Here's how the part is built. I have some questions about the finished solid (model axes, mm). Face numbers are marked on the shaded views. A direction names the side the tool comes from. Round coordinates to 2 decimals unless told otherwise and drop trailing zeros. Order: outer loops, then holes, each group sorted by start corner. A loop starts at its lowest first (then second) coordinate and runs counter-clockwise, first axis right, second up. Notation, with made-up numbers: (50, 66.5) -> (73, 66.5) arc R23 cw to (73, 96.5) -> close; hole circle Ø7 at (48, 18). An arc over 180 degrees is marked (long way). One line per item, written item: value.
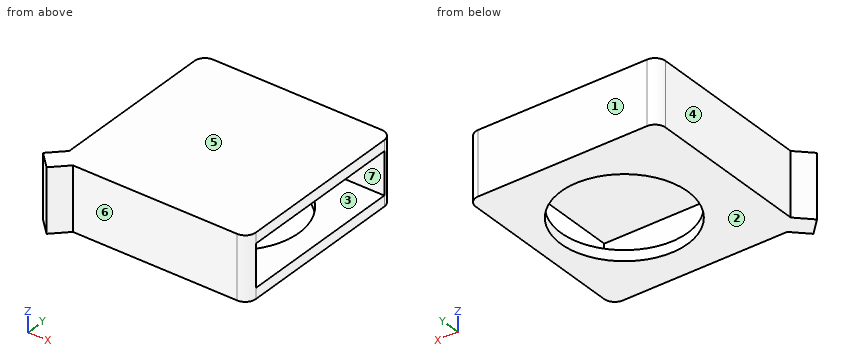
```python
from build123d import *

# Parameters (mm, degrees)
SKETCH_1_W          = 9
SKETCH_1_H          = 9
EXTRUDE_1_DEPTH     = 3
FILLET_1_R          = 0.5
SKETCH_2_R          = 3
CUT_EXTRUDE_1_DEPTH = 2.5
SKETCH_3_W          = 2
SKETCH_3_H          = 8
CUT_EXTRUDE_2_DEPTH = 8.5
EXTRUDE_2_DEPTH     = 3


with BuildPart() as part:
    # 草图1 → 凸台-拉伸1 (new body)
    with BuildSketch(Plane.XY):
        with Locations((0.284053156, -1.823920266)):
            Rectangle(SKETCH_1_W, SKETCH_1_H)
    extrude(amount=EXTRUDE_1_DEPTH)

    # 圆角1
    fillet_1_edges = [part.edges().sort_by_distance(p)[0] for p in [
        (-4.215946844, 2.676079734, 1.5),
        (4.784053156, 2.676079734, 1.5),
        (4.784053156, -6.323920266, 1.5),
        (-4.215946844, -6.323920266, 1.5),
    ]]
    fillet(fillet_1_edges, radius=FILLET_1_R)

    # 草图2 → 切除-拉伸1 (cut)
    with BuildSketch(Plane(origin=(0, 0, 0), x_dir=(-1, 0, 0), z_dir=(0, 0, -1))):
        with Locations((-0.784053156, -1.823920266)):
            Circle(SKETCH_2_R)
    extrude(amount=-CUT_EXTRUDE_1_DEPTH, mode=Mode.SUBTRACT)

    # 草图3 → 切除-拉伸2 (cut)
    with BuildSketch(Plane(origin=(4.784053156, 0, 0), x_dir=(0, 0, -1), z_dir=(1, 0, 0))):
        with Locations((-1.5, -1.823920266)):
            Rectangle(SKETCH_3_W, SKETCH_3_H)
    extrude(amount=-CUT_EXTRUDE_2_DEPTH, mode=Mode.SUBTRACT)

    # 草图4 → 凸台-拉伸2 (add)
    with BuildSketch(Plane(origin=(0, 0, 0), x_dir=(-1, 0, 0), z_dir=(0, 0, -1))):
        Polygon((4.215946844, -5.616813485), (3.508840063, -6.323920266), (4.215946844, -7.031027047), (4.923053625, -6.323920266), align=None)
    extrude(amount=-EXTRUDE_2_DEPTH)


solid = part.part
```
Q1. I want a section at D-D on x = 2. Write out the boundary of the cut face in (y, z).
Answers:
outline: (-6.32, 0) -> (-4.57, 0) -> (-4.57, 0.5) -> (-5.82, 0.5) -> (-5.82, 2.5) -> (2.18, 2.5) -> (2.18, 0.5) -> (0.92, 0.5) -> (0.92, 0) -> (2.68, 0) -> (2.68, 3) -> (-6.32, 3) -> close
Q2. I want a section at C-C on y = -1.25. Write out the boundary of the cut face in (x, z).
Answers:
outline: (-4.22, 0) -> (-2.16, 0) -> (-2.16, 0.5) -> (-3.72, 0.5) -> (-3.72, 2.5) -> (4.78, 2.5) -> (4.78, 3) -> (-4.22, 3) -> close; (3.73, 0) -> (4.78, 0) -> (4.78, 0.5) -> (3.73, 0.5) -> close
Q3. For P1, Ø0.6, axis at y = -3, z = 1.5, coming from the +X side; P2, Ø0.9, axis at x = 0.5, z = 2, coming from the -Y side, each with a flat end and sliding along its axis, tell me the tip position at first contact or that it passes through.
Answers:
P1: x = -3.72
P2: y = -6.32
Q4. Which directions (+Z, -Z, +X, -X, +Y, -Y) give clear straight access to the entire face, cutting with the end or side of a thin tool? Please do the marked faces 4, 5, 6 and 7.
Answers:
face 4: +Z, -Z, -X, +Y
face 5: +Z, +X, -X, +Y, -Y
face 6: +Z, -Z, +X, -Y
face 7: +X
Q5. I want a section at B-B on z = 2.1. Write out the boundary of the cut face in (x, y).
Answers:
outline: (-4.92, -6.32) -> (-4.22, -7.03) -> (-3.51, -6.32) -> (4.28, -6.32) arc R0.5 ccw to (4.78, -5.82) -> (-3.72, -5.82) -> (-3.72, 2.18) -> (4.78, 2.18) arc R0.5 ccw to (4.28, 2.68) -> (-3.72, 2.68) arc R0.5 ccw to (-4.22, 2.18) -> (-4.22, -5.62) -> close
Q6. I want a section at A-A on x = -2.75. Write out the boundary of the cut face in (y, z), then the cut area to 3 significant figures.
Answers:
outline: (-6.32, 0) -> (2.68, 0) -> (2.68, 3) -> (-6.32, 3) -> close; hole (-5.82, 0.5) -> (2.18, 0.5) -> (2.18, 2.5) -> (-5.82, 2.5) -> close
area: 11.0 mm2
Q7. I need wall thicknesses on line 1 along Y through (x, z) = (0.5, 2.25); line 2 along Z through (x, y) = (2.25, -4.75); line 3 along Z through (x, y) = (-0.5, 0.25). Which ranges of each line are inside material? Lowest first, please.
Answers:
line 1: -6.32 to -5.82, 2.18 to 2.68
line 2: 0 to 0.5, 2.5 to 3
line 3: 2.5 to 3
Q8. If we mould it in two halves opening along Z, with no side actions, what happens to the marked faces 1, 2 and 3? For each: pulls with the +Z half, pulls with the -Z half, needs draft (parallel to the pull), parting line crosses it, or undercut.
Answers:
face 1: needs draft
face 2: pulls with the -Z half
face 3: undercut
